Geometry check sheet. Reference: the model listing, model coordinates, mm. Coordinates: 2 decimals unless noted, no trailing zeros. Write each loop counter-clockwise with the first axis right and the second up, starting at its lowest first coordinate (ties: lowest second). Pieces come first, ordered by that corner, then holes. Notation, with made-up numbers: (31, 7) -> (68, 7) arc R16 ccw to (68, 34) -> close; hole circle Ø6 at (-30, -37). An arc over 180 degrees is marked (long way). Answer in a Markdown table with one row per item. Add a question column.
1. Cross-section at D-D on x = 8.5. Record the cut outline in (y, z).
2. Scan lines: L1, parallel to Z at x = 0.5, y = 9.25; L2, parallel to Z at x = 1, y = 5.75; L3, parallel to X at y = 6.25, z = 3.5. Record each from-to range of solid material in increasing order. Write a range as from..to.
3. Mould release check, pull along X, two halves, no side actions. Record for faces 1 (the cylindrical face through (11.66, 5.07, 12.68)), 2 (the cylindrical face through (-0.371, 4.93, 8.927)), 3 (the cylindrical face through (-2.365, 4.93, -17.412)): pulls with the +X half, pulls with the -X half, needs draft (parallel to the pull), parting line crosses it, or undercut.
4. Cross-section at A-A on y = 7. Record the cut outline in (x, z).
5. Depth check by flat-ended pin: P1, Ø2, axis at x = -6.5, y = 6, coming from the -Z side; P2, Ø3, axis at x = -4.5, z = -9.5, coming from the +Y side; P3, Ø3, axis at y = 2.5, z = 11, coming from the -X side. Enter the tip coordinate at first touch or a pass-through.
6. Cross-section at B-B on x = -9.5. Record the cut outline in (y, z), and give its area (3 significant figures).
7. Cross-section at C-C on z = 4. Record the cut outline in (x, y), and give its area (4 significant figures).
```python
from build123d import *

# Parameters (mm, degrees)
BOSS_EXTRUDE2_DEPTH = 10
FILLET1_R           = 5


with BuildPart() as part:
    # Sketch1 → Boss-Extrude2 (new body)
    with BuildSketch(Plane(origin=(0, 0, 0), x_dir=(1, 0, 0), z_dir=(0, 1, 0))):
        with BuildLine():
            ThreePointArc((-13.512538708, 1.615980507), (-2.712538708, 12.415980507), (8.087461292, 1.615980507))
            Line((8.087461292, 1.615980507), (13.087461292, 1.615980507))
            ThreePointArc((13.087461292, 1.615980507), (-2.712538708, 17.415980507), (-18.512538708, 1.615980507))
            Line((-18.512538708, 1.615980507), (-13.512538708, 1.615980507))
        make_face()
        with BuildLine():
            Line((13.087461292, 1.615980507), (8.087461292, 1.615980507))
            ThreePointArc((8.087461292, 1.615980507), (-2.712538708, -9.184019493), (-13.512538708, 1.615980507))
            Line((-13.512538708, 1.615980507), (-18.512538708, 1.615980507))
            ThreePointArc((-18.512538708, 1.615980507), (-13.884825857, -9.55630663), (-2.712538726, -14.184019493))
            ThreePointArc((-2.712538726, -14.184019493), (8.459748429, -9.556306643), (13.087461292, 1.615980507))
        make_face()
        with BuildLine():
            Line((13.087461292, -14.184019493), (13.087461292, 1.615980507))
            ThreePointArc((13.087461292, 1.615980507), (8.459748429, -9.556306643), (-2.712538726, -14.184019493))
            Line((-2.712538726, -14.184019493), (13.087461292, -14.184019493))
        make_face()
        with BuildLine():
            ThreePointArc((-2.712538726, -14.184019493), (-13.884825857, -9.55630663), (-18.512538708, 1.615980507))
            Line((-18.512538708, 1.615980507), (-18.512538708, -14.184019493))
            Line((-18.512538708, -14.184019493), (-2.712538726, -14.184019493))
        make_face()
    extrude(amount=BOSS_EXTRUDE2_DEPTH)

    # Fillet1
    fillet1_edges = [part.edges().sort_by_distance(p)[0] for p in [
        (13.087461292, 5, 14.184019493),
        (-18.512538708, 5, 14.184019493),
    ]]
    fillet(fillet1_edges, radius=FILLET1_R)


solid = part.part
```
Results found:
| question | item | result |
|---|---|---|
| 1 | outline | (0, -12.75) -> (10, -12.75) -> (10, 14.17) -> (0, 14.17) -> close |
| 2 | L1 | z = -17.09..-11.93, 8.7..14.18 |
| 2 | L2 | z = -16.97..-11.76, 8.53..14.18 |
| 2 | L3 | x = -18.51..-12.22, 6.8..13.09 |
| 3 | face 1 | pulls with the +X half |
| 3 | face 2 | undercut |
| 3 | face 3 | parting line crosses it |
| 4 | outline | (-18.51, -1.62) arc R15.8 ccw to (13.09, -1.62) -> (13.09, 9.18) arc R5 ccw to (8.09, 14.18) -> (-13.51, 14.18) arc R5 ccw to (-18.51, 9.18) -> close; hole circle Ø21.6 at (-2.71, -1.62) |
| 5 | P1 | stops at z = -17.17 |
| 5 | P2 | passes through |
| 5 | P3 | stops at x = -18.5 |
| 6 | outline | (0, -15.88) -> (10, -15.88) -> (10, -10.02) -> (0, -10.02) -> close; (0, 6.78) -> (10, 6.78) -> (10, 14.18) -> (0, 14.18) -> close |
| 6 | area | 133 mm^2 |
| 7 | outline | (-18.51, 0) -> (-11.94, 0) -> (-11.94, 10) -> (-18.51, 10) -> close; (6.51, 0) -> (13.09, 0) -> (13.09, 10) -> (6.51, 10) -> close |
| 7 | area | 131.5 mm^2 |
